Build history of the part. All positions in model axes, mm. A direction names the side the tool comes from. Coordinates: 2 decimals unless noted, no trailing zeros. Write each loop counter-clockwise with the first axis right and the second up, starting at its lowest first coordinate (ties: lowest second). Pieces come first, ordered by that corner, then holes.
```python
from build123d import *

# Parameters (mm, degrees)
SKETCH1_W           = 58.42
SKETCH1_H           = 58.42
BOSS_EXTRUDE1_DEPTH = 33.02
CUT_EXTRUDE1_DEPTH  = 30.600000014
SKETCH3_W           = 16.5
SKETCH3_H           = 9
CUT_EXTRUDE2_DEPTH  = 30.600000014


with BuildPart() as part:
    # Sketch1 → Boss-Extrude1 (new body)
    with BuildSketch(Plane(origin=(0, 0, 0), x_dir=(1, 0, 0), z_dir=(0, 1, 0))):
        with Locations((29.21, 29.21)):
            Rectangle(SKETCH1_W, SKETCH1_H)
    extrude(amount=BOSS_EXTRUDE1_DEPTH)

    # Sketch2 → Cut-Extrude1 (cut)
    with BuildSketch(Plane(origin=(0, 33.02, 0), x_dir=(1, 0, 0), z_dir=(0, 1, 0))):
        Polygon((11.495533906, 50.46), (46.924466094, 50.46), (50.46, 46.924466094), (50.46, 37.46), (57.26, 37.46), (57.26, 20.96), (50.46, 20.96), (50.46, 11.495533906), (46.924466094, 7.96), (11.495533906, 7.96), (7.96, 11.495533906), (7.96, 46.924466094), align=None)
    extrude(amount=-CUT_EXTRUDE1_DEPTH, mode=Mode.SUBTRACT)

    # Sketch3 → Cut-Extrude2 (cut)
    with BuildSketch(Plane(origin=(58.42, 0, 0), x_dir=(0, 0, -1), z_dir=(1, 0, 0))):
        with Locations((29.21, 6.919999986)):
            Rectangle(SKETCH3_W, SKETCH3_H)
    extrude(amount=-CUT_EXTRUDE2_DEPTH, mode=Mode.SUBTRACT)


solid = part.part
```
1. Saw through at C-C on y = 10.5. List the corners of the cut face in (x, z), plus the area to 3 significant figures.
Computed values:
outline: (0, -58.42) - (58.42, -58.42) - (58.42, -37.46) - (50.46, -37.46) - (50.46, -46.92) - (46.92, -50.46) - (11.5, -50.46) - (7.96, -46.92) - (7.96, -11.5) - (11.5, -7.96) - (46.92, -7.96) - (50.46, -11.5) - (50.46, -20.96) - (58.42, -20.96) - (58.42, 0) - (0, 0) - close
area: 1,500 mm2
2. Saw through at B-B on y = 14. List the corners of the cut face in (x, z).
Computed values:
outline: (0, -58.42) - (58.42, -58.42) - (58.42, 0) - (0, 0) - close; hole (7.96, -46.92) - (11.5, -50.46) - (46.92, -50.46) - (50.46, -46.92) - (50.46, -37.46) - (57.26, -37.46) - (57.26, -20.96) - (50.46, -20.96) - (50.46, -11.5) - (46.92, -7.96) - (11.5, -7.96) - (7.96, -11.5) - close
3. Flat gauge pin, fed straight in: pin 1 (1.5 mm diameter, centred on x = 27, z = -42.5, fed in from +Y). Where does the tip first touch, or does it go through?
Computed values:
pin 1: stops at y = 2.42
4. Mould opens along Z. For faces 3 (the face through (58.42, 16, -29)), 4 (the face through (48.717, 17.934, -9.753)), 5 (the face through (57.26, 22, -29)), 6 (the face through (29, 16, -58.42)) say: +Z half, -Z half, draft (parallel to the pull), parting line (faces both ways), or undercut.
Computed values:
face 3: draft
face 4: undercut
face 5: undercut
face 6: -Z half
5. Saw through at D-D on x = 36.5. List the corners of the cut face in (y, z), plus the area to 3 significant figures.
Computed values:
outline: (0, -58.42) - (33.02, -58.42) - (33.02, -50.46) - (2.42, -50.46) - (2.42, -7.96) - (33.02, -7.96) - (33.02, 0) - (0, 0) - close
area: 629 mm2
6. Saw through at A-A on z = -30.5. List the corners of the cut face in (x, y), plus the area to 3 significant figures.
Computed values:
outline: (0, 0) - (58.42, 0) - (58.42, 2.42) - (7.96, 2.42) - (7.96, 33.02) - (0, 33.02) - close; (57.26, 11.42) - (58.42, 11.42) - (58.42, 33.02) - (57.26, 33.02) - close
area: 410 mm2
7. 3-axis set-ups, long thin cutter, end or side, ignore diameter. For faces 1 (the face through (29, 0, -30)), 2 (the face through (9.753, 17.934, -9.703)): which of +Z, -Z, +X, -X, +Y, -Y reach the whole face in a straight line?
Computed values:
face 1: +Z, -Z, +X, -X, -Y
face 2: +Y
8. Probe line 1 along Z through (x, y) = (18, 17.5); line 2 along X through (y, z) = (14, -36); line 3 along X through (y, z) = (10.5, -45.5). List the from-to ranges inside material, lowest first.
Computed values:
line 1: z = -58.42 to -50.46, -7.96 to 0
line 2: x = 0 to 7.96, 57.26 to 58.42
line 3: x = 0 to 7.96, 50.46 to 58.42
